Design review of the part shown in the three views and the two pictorial views. Dimensions are in mm from the part's minimum x, y and z. Coordinates: 2 decimals unless noted, no trailing zeros. Write each loop counter-clockwise with the first axis right and the second up, starting at its lowest first coordinate (ties: lowest second). Pieces come first, ordered by that corner, then holes.
Q1. Take a section at A-A, the plane x = 10.5. Write out the cut boundary in (y, z).
Q2. Take a section at C-C, the plane x = 16. Write out the cut boundary in (y, z), plus the area to 3 significant figures.
Q3. Take a section at D-D, the plane z = 0.4. Write out the cut boundary in (x, y), plus the area to 3 significant figures.
Q4. Take a section at B-B, the plane y = 10.5. Write out the cut boundary in (x, z).
Q5. The part is to be moulded in two halves that separate along X. For the marked faces 1, 2 and 3, say which applies: released by +X, released by -X, zero draft, split by the parting line, or undercut.
Q6. For pin 1 Ø1.5 at (y, z) = (14, 2.5) entering from +X, flat-tipped, find the tip position at first contact; note if it passes through.
Q7. For L1, parallel to Y at x = 10.5, z = 2.85; L2, parallel to X at y = 6.5, z = 3.1; L3, parallel to X at y = 20.2, z = 1.75, list the stretches that pass through material, from the lowest coordinate up.
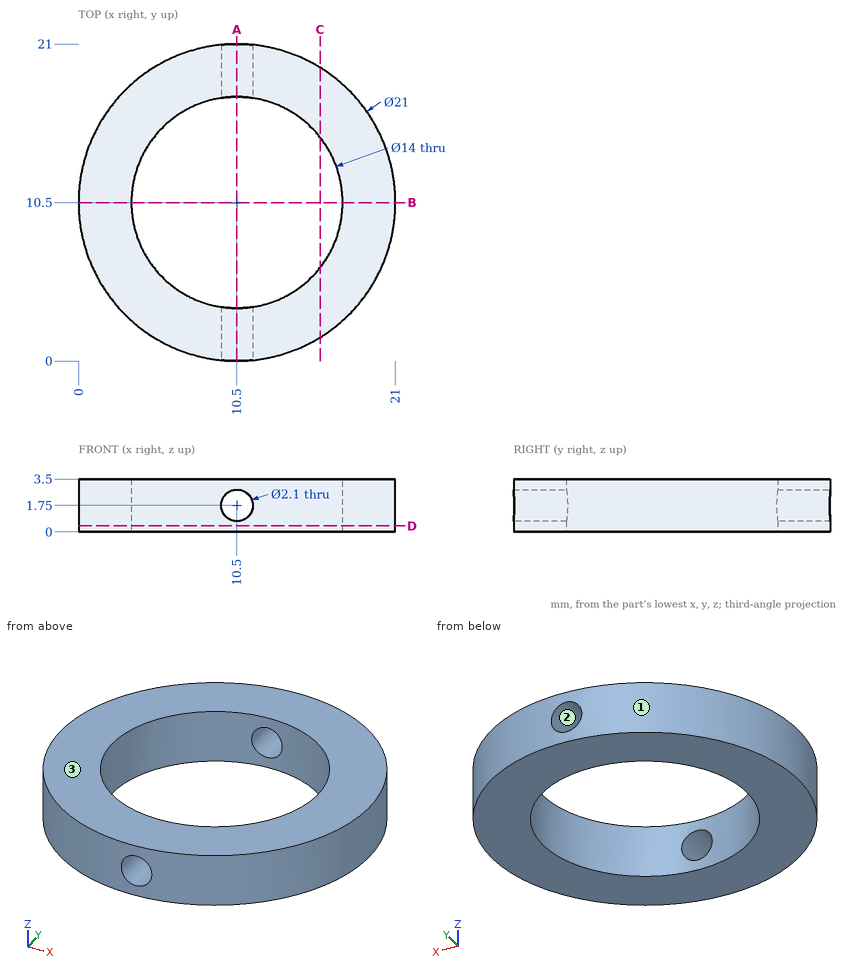
Responses:
1. outline: (0, 0) - (3.5, 0) - (3.5, 0.7) - (0, 0.7) - close; (0, 2.8) - (3.5, 2.8) - (3.5, 3.5) - (0, 3.5) - close; (17.5, 0) - (21, 0) - (21, 0.7) - (17.5, 0.7) - close; (17.5, 2.8) - (21, 2.8) - (21, 3.5) - (17.5, 3.5) - close
2. outline: (1.56, 0) - (6.17, 0) - (6.17, 3.5) - (1.56, 3.5) - close; (14.83, 0) - (19.44, 0) - (19.44, 3.5) - (14.83, 3.5) - close
2. area: 32.3 mm2
3. outline: circle Ø21 at (10.5, 10.5); hole circle Ø14 at (10.5, 10.5)
3. area: 192 mm2
4. outline: (0, 0) - (3.5, 0) - (3.5, 3.5) - (0, 3.5) - close; (17.5, 0) - (21, 0) - (21, 3.5) - (17.5, 3.5) - close
5. face 1: split by the parting line
5. face 2: undercut
5. face 3: zero draft
6. pin 1: stops at x = 20.63
7. L1: y = 0 to 3.5, 17.5 to 21
7. L2: x = 0.79 to 4.76, 16.24 to 20.21
7. L3: x = 6.48 to 9.45, 11.55 to 14.52
